```python
from build123d import *

# Parameters (mm, degrees)
F1_DEPTH = 12
F0_R     = 2
F2_DEPTH = 8
F3_SIZE  = 1
F4_R     = 4.15
F5_DEPTH = 8
F6_R     = 3
F7_DEPTH = 3


with BuildPart() as f1:
    # F0 (on Top) → F1 (new body)
    with BuildSketch(Plane.XY):
        Polygon((14.7, 8.5), (-14.7, 8.5), (-19, 4.2), (-19, -4.2), (-14.7, -8.5), (14.7, -8.5), (19, -4.2), (19, 4.2), align=None)
    extrude(amount=F1_DEPTH)

    # F0 (on Top) → F2 (join)
    with BuildSketch(Plane.XY):
        Polygon((22.5, 11.5), (-22.5, 11.5), (-28.5, 5.5), (-28.5, -5.5), (-22.5, -11.5), (22.5, -11.5), (28.5, -5.5), (28.5, 5.5), align=None)
        with Locations((-24.75, 0)):
            Circle(F0_R, mode=Mode.SUBTRACT)
        Polygon((-19, 4.2), (-14.7, 8.5), (14.7, 8.5), (19, 4.2), (19, -4.2), (14.7, -8.5), (-14.7, -8.5), (-19, -4.2), align=None, mode=Mode.SUBTRACT)
        with Locations((24.75, 0)):
            Circle(F0_R, mode=Mode.SUBTRACT)
    extrude(amount=F2_DEPTH)

    # F3
    f3_edges = [f1.edges().sort_by_distance(p)[0] for p in [
        (0, -11.5, 0),
        (-25.5, -8.5, 0),
        (-28.5, 0, 0),
        (-25.5, 8.5, 0),
        (0, 11.5, 0),
        (25.5, 8.5, 0),
        (28.5, 0, 0),
        (25.5, -8.5, 0),
    ]]
    chamfer(f3_edges, length=F3_SIZE)

    # F4 (on face) → F5 (cut)
    with BuildSketch(Plane.XY.offset(12)):
        Circle(F4_R)
    extrude(amount=-F5_DEPTH, mode=Mode.SUBTRACT)

    # F6 (on Top) → F7 (cut)
    with BuildSketch(Plane.XY):
        with Locations((-23.793586, 0)):
            Circle(F6_R)
        with Locations((23.756452, 0)):
            Circle(F6_R)
    extrude(amount=F7_DEPTH, mode=Mode.SUBTRACT)


solid = f1.part
```
Source: CAD feature listing. Evaluate the final solid. Frame: model axes, mm. A direction names the side the tool comes from. Round coordinates to 2 decimals unless told otherwise and drop trailing zeros. Loops run counter-clockwise (first coordinate to the right, second up) from the corner with the lowest first, then second, coordinate; pieces in that order, holes last. Notation, with made-up numbers: M -1.75,45 L 2.25,45 A18 ccw 2.25,69 Z; hole C 33,-18 d6. An arc over 180 degrees is marked long. Use a Markdown table: item, result. Add a question column.
1. Cut plane D-D, the plane x = 10. Output: boundary loops of the cut face in (y, z).
2. Cut plane B-B, the plane x = 24.75. Output: boundary loops of the cut face in (y, z), and give its area (3 significant figures).
3. Contact query for flat-ended pins moving along their axis: pin 1 (4.5 mm diameter, centred on x = 3, z = 10.5, fed in from +Y); pin 2 (1.8 mm diameter, centred on x = -23.5, y = 0, fed in from -Z); pin 3 (1.2 mm diameter, centred on y = 1, z = 10, fed in from +X). Output: stop coordinate, or through.
4. Pull-direction query (X, two-part tool) for faces 5 (the flat face through (26, 8, 4)), 6 (the flat face through (0.3, 11, 0.5)), 7 (the flat face through (0, 0, 4)), 8 (the flat face through (-25.193, -8.109, 0.507)); classes: +X half, -X half, draft (parallel to the pull), parting line (faces both ways), or undercut.
5. Set-up query: faces 1 (the flat face through (0, -10, 8)), 2 (the flat face through (-19, 0, 10)), 3 (the cylindrical face through (-26.79, 0.13, 1.48)), 4 (the flat face through (-16.9, -6.3, 10)). Return all of +Z, -Z, +X, -X, +Y, -Y with unobstructed straight access to the full face (end or side cutting, diameter ignored); none if empty.
6. Cut plane A-A, the plane y = 0. State how many separate pieces and enclosed holes the cut face has, and give its area (3 significant figures).
7. Cut plane C-C, the plane z = 8.75. Output: boundary loops of the cut face in (x, y).
8. Ray query, line 1 along Y through (x, z) = (5, 11.5); line 2 along Y through (x, z) = (-24.75, 6.4); line 3 along Z through (x, y) = (25.5, 6.75). Return the intervals inside material, ascending. Write a range as [from, to].
Solution:
| question | item | result |
|---|---|---|
| 1 | outline | M -11.5,1 L -10.5,0 L 10.5,0 L 11.5,1 L 11.5,8 L 8.5,8 L 8.5,12 L -8.5,12 L -8.5,8 L -11.5,8 Z |
| 2 | outline | M -9.25,1 L -7.84,0 L -2.83,0 L -2.83,3 L -2,3 L -2,8 L -9.25,8 Z; M 2,3 L 2.83,3 L 2.83,0 L 7.84,0 L 9.25,1 L 9.25,8 L 2,8 Z |
| 2 | area | 110 mm2 |
| 3 | pin 1 | stops at y = 8.5 |
| 3 | pin 2 | stops at z = 3 |
| 3 | pin 3 | stops at x = 19 |
| 4 | face 5 | +X half |
| 4 | face 6 | draft |
| 4 | face 7 | undercut |
| 4 | face 8 | -X half |
| 5 | face 1 | +Z |
| 5 | face 2 | +Z, -X, +Y, -Y |
| 5 | face 3 | -Z |
| 5 | face 4 | +Z, -X, -Y |
| 6 | separate pieces | 3 |
| 6 | enclosed holes | 0 |
| 6 | area | 465 mm2 |
| 7 | outline | M -19,-4.2 L -14.7,-8.5 L 14.7,-8.5 L 19,-4.2 L 19,4.2 L 14.7,8.5 L -14.7,8.5 L -19,4.2 Z; hole C 0,0 d8.3 |
| 8 | line 1 | y = [-8.5, 8.5] |
| 8 | line 2 | y = [-9.25, -2], [2, 9.25] |
| 8 | line 3 | z = [0, 8] |
